from build123d import *

# Parameters (mm, degrees)
F1_DEPTH = 1.27
F2_R     = 0.635
F4_D     = 3.81


with BuildPart() as f1:
    # F0 (on Front) → F1 (new body)
    with BuildSketch(Plane.XZ):
        with BuildLine():
            ThreePointArc((-3.175, -2.54), (-1.378949, -1.796051), (-0.635, 0))
            ThreePointArc((-0.635, 0), (-1.378949, 1.796051), (-3.175, 2.54))
            ThreePointArc((-3.175, 2.54), (-5.715, 0), (-3.175, -2.54))
        make_face()
        with BuildLine():
            ThreePointArc((-3.175, 2.54), (-1.378949, 1.796051), (-0.635, 0))
            ThreePointArc((-0.635, 0), (-1.378949, -1.796051), (-3.175, -2.54))
            Line((-3.175, -2.54), (3.175, -2.54))
            ThreePointArc((3.175, -2.54), (0.635, 0), (3.175, 2.54))
            Line((3.175, 2.54), (-3.175, 2.54))
        make_face()
        with BuildLine():
            ThreePointArc((5.715, 0), (4.971051, 1.796051), (3.175, 2.54))
            ThreePointArc((3.175, 2.54), (0.635, 0), (3.175, -2.54))
            ThreePointArc((3.175, -2.54), (4.971051, -1.796051), (5.715, 0))
        make_face()
    extrude(amount=F1_DEPTH)

    # F2
    f2_edges = [f1.edges().sort_by_distance(p)[0] for p in [
        (0, 0, -2.54),
    ]]
    fillet(f2_edges, radius=F2_R)

    # F4 (through all)
    with Locations(Plane.XZ.offset(1.27)):
        with Locations((3.175, 0)):
            Hole(F4_D / 2)


solid = f1.part
Verification items for the finished model (mm, model axes). Coordinates: 2 decimals unless noted, no trailing zeros. Order: outer loops, then holes, each group sorted by start corner. A loop starts at its lowest first (then second) coordinate and runs counter-clockwise, first axis right, second up. Notation, with made-up numbers: M 83,-23.5 L 94,-23.5 A34 ccw 94,9.5 Z; hole C 29,-23 d8. An arc over 180 degrees is marked long. One line per item, written item: value. Start each with the question number.
Item 1: Sectioned sample at B-B (x = 1.5). Enter the section's corners in (y, z) (3 decimals), then the cut area to 3 significant figures.
Item 2: Sectioned sample at C-C (x = -2.5). Enter the section's corners in (y, z) (3 decimals).
Item 3: Sectioned sample at D-D (y = -0.45). Enter the section's corners in (x, z) (3 decimals).
Item 4: Scan lines: probe 1 along Z at (x, y) = (3.25, -1.05); probe 2 along X at (y, z) = (-0.35, 0.75); probe 3 along X at (y, z) = (-0.2, -0.25). Record each from-to range of solid material in increasing order.
Item 5: Sectioned sample at A-A (y = -1.1). Enter the section's corners in (x, z) (3 decimals).
Item 6: Mould release check, pull along Z, two halves, no side actions. Record for faces 1 (the cylindrical face through (-5.714, -0.948, 0.056)), 2 (the cylindrical face through (1.358, -0.626, 0.572)), 3 (the flat face through (-2, 0, 0)): released by +Z, released by -Z, zero draft, split by the parting line, or undercut.
Conclusion:
1. outline: M -1.27,-2.54 L -0.635,-2.54 A0.635 ccw 0,-1.905 L 0,-0.907 L -1.27,-0.907 Z; M -1.27,0.907 L 0,0.907 L 0,1.905 A0.635 ccw -0.635,2.54 L -1.27,2.54 Z
1. area: 3.97 mm^2
2. outline: M -1.27,-2.54 L -0.635,-2.54 A0.635 ccw 0,-1.905 L 0,1.905 A0.635 ccw -0.635,2.54 L -1.27,2.54 Z
3. outline: M -3.175,-2.512 L 3.175,-2.512 A2.512 ccw 5.687,0 A2.512 ccw 3.175,2.512 L -3.175,2.512 A2.512 ccw Z; hole C 3.175,0 d3.81
4. probe 1: z = -2.54 to -1.9, 1.9 to 2.54
4. probe 2: x = -5.53 to 1.42, 4.93 to 5.53
4. probe 3: x = -5.53 to 1.29, 5.06 to 5.53
5. outline: M -3.175,-2.54 L 3.175,-2.54 A2.54 ccw 5.715,0 A2.54 ccw 3.175,2.54 L -3.175,2.54 A2.54 ccw Z; hole C 3.175,0 d3.81
6. face 1: split by the parting line
6. face 2: undercut
6. face 3: zero draft
